For this review, take the finished solid that the model builds, in its own axes (mm). A direction names the side the tool comes from. Give positions to 0.01 mm unless a question says otherwise; leave off trailing zeros. Write each loop counter-clockwise with the first axis right and the second up, starting at its lowest first coordinate (ties: lowest second). Pieces come first, ordered by that corner, then holes. Notation, with made-up numbers: (-23.5, 51) -> (-2.5, 51) arc R18 cw to (-2.5, 59) -> close; hole circle Ø9 at (61.25, 22). An arc over 180 degrees is marked (long way). Answer as CSV lines item,"result".
```python
from build123d import *

# Parameters (mm, degrees)
SKETCH_4_R      = 10
EXTRUDE_4_DEPTH = 30
SKETCH_5_R      = 10
EXTRUDE_5_DEPTH = 28
SKETCH_6_R      = 15
EXTRUDE_6_DEPTH = 5
EXTRUDE_START   = 92
SKETCH_7_R      = 10
EXTRUDE_7_DEPTH = 92
CHAMFER_2_SIZE  = 2


with BuildPart() as part:
    # 草图4 → 凸台-拉伸4 (new body)
    with BuildSketch(Plane(origin=(0, 0, 0), x_dir=(0, 0, -1), z_dir=(1, 0, 0))):
        with BuildLine():
            Line((-34.805554051, -3.684210526), (-24.861110036, -97.631578947))
            ThreePointArc((-24.861110036, -97.631578947), (0, -120), (24.861110036, -97.631578947))
            Line((24.861110036, -97.631578947), (34.805554051, -3.684210526))
            ThreePointArc((34.805554051, -3.684210526), (0, 35), (-34.805554051, -3.684210526))
        make_face()
        with Locations((0, -95)):
            Circle(SKETCH_4_R, mode=Mode.SUBTRACT)
        Polygon((0, 21.213203436), (21.213203436, 0), (0, -21.213203436), (-21.213203436, 0), align=None, mode=Mode.SUBTRACT)
    extrude(amount=-EXTRUDE_4_DEPTH)

    # 草图5 → 凸台-拉伸5 (add)
    with BuildSketch(Plane(origin=(0, 0, 0), x_dir=(0, 0, -1), z_dir=(1, 0, 0))):
        with Locations((0, -95)):
            Circle(SKETCH_5_R)
    extrude(amount=-EXTRUDE_5_DEPTH)

    # 草图6 → 凸台-拉伸6 (add)
    with BuildSketch(Plane(origin=(0, 0, 0), x_dir=(0, 0, -1), z_dir=(1, 0, 0))):
        with Locations(Location((0, -95, 0), (0, 0, 180))):
            Circle(SKETCH_6_R)
    extrude(amount=EXTRUDE_6_DEPTH)

    # 草图7 → 凸台-拉伸7 (add)
    with BuildSketch(Plane(origin=(5, 0, 0), x_dir=(0, 0, -1), z_dir=(1, 0, 0)).offset(EXTRUDE_START)):
        with Locations((0, -95)):
            Circle(SKETCH_7_R)
    extrude(amount=-EXTRUDE_7_DEPTH)

    # 倒角2
    chamfer_2_edges = [part.edges().sort_by_distance(p)[0] for p in [
        (97, -95, 10),
    ]]
    chamfer(chamfer_2_edges, length=CHAMFER_2_SIZE)


solid = part.part
```
Q1. Draft analysis for pull direction Y (two halves, no side actions). For faces 4 (the cylindrical face through (-14.79, -119.995, 0.513)), 5 (the flat face through (0, -41, 0)), 6 (the flat face through (-28, -95, 0)), state which applies: released by +Y, released by -Y, zero draft, split by the parting line, or undercut.
Answer block:
face 4,"released by -Y"
face 5,"zero draft"
face 6,"undercut"
Q2. Add section D-D (z = -28.5). Write out the cut boundary in (x, y).
Answer block:
outline,"(-30, -63.25) -> (0, -63.25) -> (0, 20.32) -> (-30, 20.32) -> close"
Q3. For faces 1 (the flat face through (-14.79, 10.755, -10.458)), 2 (the cylindrical face through (2.465, -80.357, -3.252)), 3 (the cylindrical face through (-28.986, -85.085, 1.302)), list the 3-axis set-ups (+Z, -Z, +X, -X, +Y, -Y) from which the entire face can be reached by the end or side of a thin tool; tool diameter is ignored.
Answer block:
face 1,"+X, -X"
face 2,"+X"
face 3,"-X"
Q4. To check wall thickness, follow probe 1 along X at (y, z) = (-56, -14); probe 2 along X at (y, z) = (-106, 0.5); probe 3 along Y at (x, z) = (-18, -16). State the ranges of each line that lie inside material, in increasing order. Write a range as [from, to].
Answer block:
probe 1,"x = [-30, 0]"
probe 2,"x = [-30, 5]"
probe 3,"y = [-114.21, -5.21], [5.21, 31.13]"
Q5. Add section A-A (y = -7). Write out the cut boundary in (x, z), plus the area to 3 significant figures.
Answer block:
outline,"(-30, -34.45) -> (0, -34.45) -> (0, -14.21) -> (-30, -14.21) -> close; (-30, 14.21) -> (0, 14.21) -> (0, 34.45) -> (-30, 34.45) -> close"
area,"1,210 mm2"
Q6. Clearance check with flat-ended pins moving along their axes: pin 1 (6 mm diameter, centred on y = -93.5, z = 2, fed in from -X); pin 2 (12 mm diameter, centred on x = 54, z = -1, fed in from +Y); pin 3 (3 mm diameter, centred on y = -42, z = -3.5, fed in from +X). State where each tip first meets the part, or that it passes through.
Answer block:
pin 1,"stops at x = -28"
pin 2,"stops at y = -85"
pin 3,"stops at x = 0"
Q7. Add section C-C (x = 65.5). Write out the cut boundary in (y, z).
Answer block:
outline,"circle Ø20 at (-95, 0)"
Q8. Add section B-B (y = -95). Write out the cut boundary in (x, z), plus the area to 3 significant figures.
Answer block:
outline,"(-30, -25.14) -> (0, -25.14) -> (0, -15) -> (5, -15) -> (5, -10) -> (95, -10) -> (97, -8) -> (97, 8) -> (95, 10) -> (5, 10) -> (5, 15) -> (0, 15) -> (0, 25.14) -> (-30, 25.14) -> (-30, 10) -> (-28, 10) -> (-28, -10) -> (-30, -10) -> close"
area,"3,450 mm2"
